Source: CAD feature listing. Evaluate the final solid. Frame: model axes, mm. Face numbers are marked on the shaded views. A direction names the side the tool comes from. Coordinates: 2 decimals unless noted, no trailing zeros. Order: outer loops, then holes, each group sorted by start corner. A loop starts at its lowest first (then second) coordinate and runs counter-clockwise, first axis right, second up.
```python
from build123d import *

# Parameters (mm, degrees)
SKETCH1_R           = 1.75
BOSS_EXTRUDE1_DEPTH = 1.6
SKETCH2_W           = 4
SKETCH2_H           = 5
BOSS_EXTRUDE2_DEPTH = 1.6
SKETCH3_R           = 5
BOSS_EXTRUDE3_DEPTH = 1


with BuildPart() as part:
    # Sketch1 → Boss-Extrude1 (new body)
    with BuildSketch(Plane(origin=(0, 0, 0), x_dir=(1, 0, 0), z_dir=(0, 1, 0))):
        with BuildLine():
            Line((-9.5, -11.5), (9.5, -11.5))
            ThreePointArc((9.5, -11.5), (10.914213562, -10.914213562), (11.5, -9.5))
            Line((11.5, -9.5), (11.5, 9.5))
            ThreePointArc((11.5, 9.5), (10.914213562, 10.914213562), (9.5, 11.5))
            Line((9.5, 11.5), (-9.5, 11.5))
            ThreePointArc((-9.5, 11.5), (-10.914213562, 10.914213562), (-11.5, 9.5))
            Line((-11.5, 9.5), (-11.5, -9.5))
            ThreePointArc((-11.5, -9.5), (-10.914213562, -10.914213562), (-9.5, -11.5))
        make_face()
        with Locations((8.5, 8.5)):
            Circle(SKETCH1_R, mode=Mode.SUBTRACT)
        with Locations((8.5, -8.5)):
            Circle(SKETCH1_R, mode=Mode.SUBTRACT)
        with Locations((-8.5, -8.5)):
            Circle(SKETCH1_R, mode=Mode.SUBTRACT)
        with Locations((-8.5, 8.5)):
            Circle(SKETCH1_R, mode=Mode.SUBTRACT)
    extrude(amount=BOSS_EXTRUDE1_DEPTH)

    # Sketch2 → Boss-Extrude2 (add)
    with BuildSketch(Plane(origin=(0, 1.6, 0), x_dir=(1, 0, 0), z_dir=(0, 1, 0))):
        Rectangle(SKETCH2_W, SKETCH2_H)
    extrude(amount=BOSS_EXTRUDE2_DEPTH)

    # Sketch3 → Boss-Extrude3 (add)
    with BuildSketch(Plane(origin=(0, 1.6, 0), x_dir=(1, 0, 0), z_dir=(0, 1, 0))):
        Circle(SKETCH3_R)
    extrude(amount=BOSS_EXTRUDE3_DEPTH)


solid = part.part
```
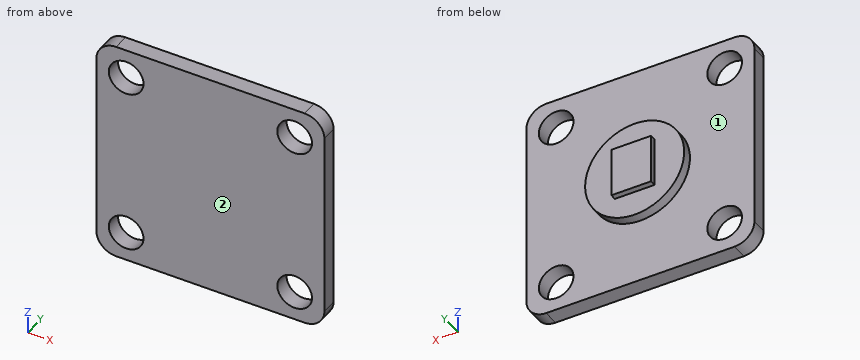
1. Pin query (flat end, axial travel): P1, Ø3, axis at x = 2, z = -3, coming from the -Y side; P2, Ø0.7, axis at y = 3, z = 0.5, coming from the +X side; P3, Ø1, axis at x = -8.5, z = 7, coming from the +Y side; P4, Ø2, axis at x = 8.5, z = -8.5, coming from the +Y side. Return the tip coordinate at first contact, or that it passes through.
Findings:
P1: stops at y = 0
P2: stops at x = 2
P3: stops at y = 1.6
P4: passes through
2. Section query D-D on x = 4. Return loops of the section in (y, z), plus the area to 3 significant figures.
Findings:
outline: (0, -11.5) - (1.6, -11.5) - (1.6, -3) - (2.6, -3) - (2.6, 3) - (1.6, 3) - (1.6, 11.5) - (0, 11.5) - close
area: 42.8 mm2
3. Access query for the marked faces 1 and 2. Directions: +Z, -Z, +X, -X, +Y, -Y. A direction counts if a zero-diameter tool reaches every point of the face in a straight line with its end or side. Return the directions, or none.
Findings:
face 1: +Y
face 2: +Z, -Z, +X, -X, -Y
4. Ray query, line 1 (X direction, y = 1.15, z = 8.5); line 2 (X direction, y = 0.45, z = -7). Return the intervals inside material, ascending.
Findings:
line 1: x = -11.5 to -10.25, -6.75 to 6.75, 10.25 to 11.5
line 2: x = -11.5 to -9.4, -7.6 to 7.6, 9.4 to 11.5
5. Section query A-A on x = -8.5. Return loops of the section in (y, z), plus the area to 3 significant figures.
Findings:
outline: (0, -11.5) - (1.6, -11.5) - (1.6, -10.25) - (0, -10.25) - close; (0, -6.75) - (1.6, -6.75) - (1.6, 6.75) - (0, 6.75) - close; (0, 10.25) - (1.6, 10.25) - (1.6, 11.5) - (0, 11.5) - close
area: 25.6 mm2
6. Section query C-C on z = -8.5. Return loops of the section in (x, y), plus the area to 3 significant figures.
Findings:
outline: (-11.5, 0) - (-10.25, 0) - (-10.25, 1.6) - (-11.5, 1.6) - close; (-6.75, 0) - (6.75, 0) - (6.75, 1.6) - (-6.75, 1.6) - close; (10.25, 0) - (11.5, 0) - (11.5, 1.6) - (10.25, 1.6) - close
area: 25.6 mm2
7. Section query B-B on y = 0.4. Return loops of the section in (x, z), plus the area to 3 significant figures.
Findings:
outline: (-11.5, -9.5) arc R2 ccw to (-9.5, -11.5) - (9.5, -11.5) arc R2 ccw to (11.5, -9.5) - (11.5, 9.5) arc R2 ccw to (9.5, 11.5) - (-9.5, 11.5) arc R2 ccw to (-11.5, 9.5) - close; hole circle Ø3.5 at (-8.5, -8.5); hole circle Ø3.5 at (-8.5, 8.5); hole circle Ø3.5 at (8.5, -8.5); hole circle Ø3.5 at (8.5, 8.5)
area: 487 mm2
